Check sheet for the modelled part. Datum: model origin and axes. Units: mm. Face numbers are marked on the shaded views. A direction names the side the tool comes from. Round coordinates to 2 decimals unless told otherwise and drop trailing zeros. Order: outer loops, then holes, each group sorted by start corner. A loop starts at its lowest first (then second) coordinate and runs counter-clockwise, first axis right, second up. Notation, with made-up numbers: M -30.5,69 L 12.5,69 A15 cw 12.5,89 Z; hole C 0.5,7 d8. An arc over 180 degrees is marked long. One line per item, written item: value. Start each with the question number.
(1) Depth check by flat-ended pin: pin 1 Ø2 at (y, z) = (6, -6) entering from +X; pin 2 Ø1.8 at (y, z) = (-6, 6) entering from +X; pin 3 Ø1.8 at (y, z) = (-6, -6) entering from -X. Enter the tip coordinate at first touch or a pass-through.
(2) Thickness scan on L1, parallel to Z at x = 21.25, y = -6; L2, parallel to Y at x = 18, z = -6.5. Record the ranges inside material, lowest first.
(3) Cross-section at B-B, the plane y = -3.75. Enter the section's corners in (x, z).
(4) Cross-section at D-D, the plane y = 3.5. Enter the section's corners in (x, z).
(5) Cross-section at A-A, the plane x = 10.5. Enter the section's corners in (y, z), and give its area (3 significant figures).
(6) Release check for a two-part mould opening along X. For the marked faces 1, 2, 3 and 4 record: released by +X, released by -X, zero draft, split by the parting line, or undercut.
(7) Cross-section at C-C, the plane z = 0. Enter the section's corners in (x, y), and give its area (3 significant figures).
(8) Access from +Z, -Z, +X, -X, +Y, -Y to the whole of each face (thin tool, end or side, straight path). Record for the marked faces 5 and 6.
from build123d import *

# Parameters (mm, degrees)
BOSS_EXTRUDE1_DEPTH = 10
CUT_EXTRUDE1_REACH  = 35.915
SKETCH3_R           = 9
SKETCH3_R_2         = 3.1
SKETCH4_R           = 1.15
CUT_EXTRUDE2_DEPTH  = 10


with BuildPart() as part:
    # Sketch2 → Boss-Extrude1 (new, symmetric)
    with BuildSketch(Plane.XY):
        Polygon((-16, -10), (25.5, -10), (25.5, 10), (-20, 10), (-20, -5), (-16, 2.5), align=None)
    extrude(amount=BOSS_EXTRUDE1_DEPTH, both=True)

    # Sketch3 → Cut-Extrude1 (cut, up to next)
    with BuildSketch(Plane(origin=(0, 10, 0), x_dir=(1, 0, 0), z_dir=(0, 1, 0)), mode=Mode.PRIVATE) as cut_extrude1_sk1:
        with Locations(Location((10.5, 0, 0), (0, 0, 270))):
            Circle(SKETCH3_R)
    cut_extrude1_tool1 = extrude(cut_extrude1_sk1.sketch, amount=-CUT_EXTRUDE1_REACH, mode=Mode.PRIVATE) & part.part
    # Sketch3 → Cut-Extrude1 (cut, up to next)
    with BuildSketch(Plane(origin=(0, 10, 0), x_dir=(1, 0, 0), z_dir=(0, 1, 0)), mode=Mode.PRIVATE) as cut_extrude1_sk2:
        with Locations((25.5, 0)):
            Circle(SKETCH3_R_2)
    cut_extrude1_tool2 = extrude(cut_extrude1_sk2.sketch, amount=-CUT_EXTRUDE1_REACH, mode=Mode.PRIVATE) & part.part
    add(cut_extrude1_tool1.solids().sort_by_distance((10.5, 10, 0))[0], mode=Mode.SUBTRACT)
    add(cut_extrude1_tool2.solids().sort_by_distance((25.5, 10, 0))[0], mode=Mode.SUBTRACT)

    # Sketch4 → Cut-Extrude2 (cut)
    with BuildSketch(Plane(origin=(25.5, 0, 0), x_dir=(0, 0, -1), z_dir=(1, 0, 0))):
        with Locations((-6, 6)):
            Circle(SKETCH4_R)
        with Locations((-6, -6)):
            Circle(SKETCH4_R)
        with Locations((6, -6)):
            Circle(SKETCH4_R)
        with Locations((6, 6)):
            Circle(SKETCH4_R)
    extrude(amount=-CUT_EXTRUDE2_DEPTH, mode=Mode.SUBTRACT)


solid = part.part
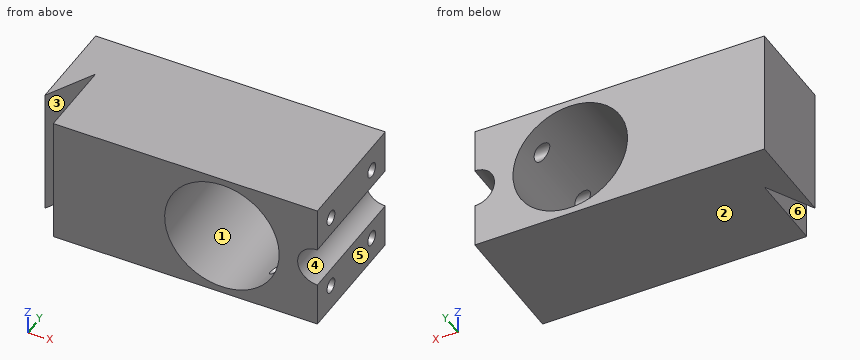
Values found:
1. pin 1: x = 4.84
1. pin 2: x = 4.72
1. pin 3: x = -16
2. L1: -10 to -7.15, -4.85 to 4.85, 7.15 to 10
2. L2: -10 to -7.04, -4.96 to 4.96, 7.04 to 10
3. outline: M -20,-10 L -19.33,-10 L -19.33,10 L -20,10 Z; M -16,-10 L 25.5,-10 L 25.5,-3.1 A3.1 cw 25.5,3.1 L 25.5,10 L -16,10 Z; hole C 10.5,0 d18
4. outline: M -20,-10 L 25.5,-10 L 25.5,-3.1 A3.1 cw 25.5,3.1 L 25.5,10 L -20,10 Z; hole C 10.5,0 d18
5. outline: M -10,-10 L 10,-10 L 10,-9 L -10,-9 Z; M -10,9 L 10,9 L 10,10 L -10,10 Z
5. area: 40.0 mm^2
6. face 1: undercut
6. face 2: zero draft
6. face 3: undercut
6. face 4: released by +X
7. outline: M -20,-5 L -16,2.5 L -16,-10 L 1.5,-10 L 1.5,10 L -20,10 Z; M 19.5,-10 L 22.4,-10 L 22.4,10 L 19.5,10 Z
7. area: 453 mm^2
8. face 5: +Z, -Z, +X, +Y, -Y
8. face 6: +Z, -Z, -Y
